```python
from build123d import *

# Parameters (mm, degrees)
F1_DEPTH = 30
F2_R     = 12
F3_DEPTH = 25
F4_R     = 14.99999
F5_DEPTH = 7.3296


# Not quite as in the source:
# - a fillet or chamfer is up to 0.001 mm smaller than in the source, because OpenCascade refuses the exact size


with BuildPart() as f1:
    # F0 (on Front) → F1 (new body)
    with BuildSketch(Plane.XZ):
        Polygon((-18.8925201073, 27.8060024955), (-18.9275150057, 27.8060024955), (-18.9275150057, 2.8060024955), (-15.9275150057, 2.8060024955), (-15.9275150057, 24.8831361532), (-10.9275150057, 24.8831361532), (-10.9275150057, 2.8060024955), (-7.9275150057, 2.8060024955), (-7.9275150057, 27.8060024955), (-10.9275150057, 27.8060024955), (-15.9275150057, 27.8060024955), (-15.9275150057, 54.8831361532), (-18.8925201073, 54.8831361532), align=None)
    extrude(amount=F1_DEPTH)

    # F2 (on face) → F3 (cut)
    with BuildSketch(Plane(origin=(-18.8925201073, 0, 0), x_dir=(0, -1, 0), z_dir=(-1, 0, 0))):
        with Locations((15, 41.3446361532)):
            Circle(F2_R)
    extrude(amount=-F3_DEPTH, mode=Mode.SUBTRACT)

    # F4 (radius 15 in the source; OpenCascade refuses exactly that, so slightly less here)
    f4_edges = [f1.edges().sort_by_distance(p)[0] for p in [
        (-17.410018, 0, 54.883136),
        (-17.410018, -30, 54.883136),
    ]]
    fillet(f4_edges, radius=F4_R)

    # F2 (on face) → F5 (cut)
    with BuildSketch(Plane(origin=(-18.8925201073, 0, 0), x_dir=(0, -1, 0), z_dir=(-1, 0, 0))):
        with Locations((15, 41.3446361532)):
            Circle(F2_R)
    extrude(amount=-F5_DEPTH, mode=Mode.SUBTRACT)


solid = f1.part
```
For this review, take the finished solid that the model builds, in its own axes (mm). A direction names the side the tool comes from. Give positions to 0.01 mm unless a question says otherwise; leave off trailing zeros.
1) The part is to be moulded in two halves that separate along Z. For faces 1 (the face through (-17.431, -4.277, 50.372)), 2 (the face through (-18.928, -15, 15)), 3 (the face through (-17.431, -13.438, 53.243)), say which applies: released by +Z, released by -Z, zero draft, split by the parting line, or undercut.
2) Insertion check: pin 1 (2 mm diameter, centred on x = -11.5, z = 15, fed in from +Y); pin 2 (6 mm diameter, centred on x = -17.5, y = -27, fed in from +Z); pin 3 (4 mm diameter, centred on x = -11, y = -10, fed in from +Z); pin 4 (2.5 mm diameter, centred on x = -14.5, y = -14, fed in from -Z). Each pin has a flat end and moves straight along its axis. Give the tip position at first contact, or say it passes through.
3) Wall thickness on line 1 (Z direction, x = -18.2, y = -15); line 2 (X direction, y = -27.5, z = 19.5); line 3 (Z direction, x = -14.25, y = -10): over which ranges is each line inside the solid? List them lowest first.
4) For faces 4 (the face through (-13, -15, 24.883)), 5 (the face through (-12, -15, 27.806)), 6 (the face through (-17, -15, 2.806)), list the 3-axis set-ups (+Z, -Z, +X, -X, +Y, -Y) from which the entire face can be reached by the end or side of a thin tool; tool diameter is ignored.
Derived:
1. face 1: released by +Z
1. face 2: zero draft
1. face 3: undercut
2. pin 1: stops at y = 0
2. pin 2: stops at z = 51.88
2. pin 3: stops at z = 27.81
2. pin 4: stops at z = 24.88
3. line 1: z = 2.81 to 29.34, 53.34 to 54.88
3. line 2: x = -18.93 to -15.93, -10.93 to -7.93
3. line 3: z = 24.88 to 27.81
4. face 4: -Z, +Y, -Y
4. face 5: +Z, +X, +Y, -Y
4. face 6: -Z, +X, -X, +Y, -Y
